Could you check a few things on this model? Use its own coordinates, in mm. A direction names the side the tool comes from. Round coordinates to 2 decimals unless told otherwise and drop trailing zeros. Order: outer loops, then holes, each group sorted by start corner. A loop starts at its lowest first (then second) coordinate and runs counter-clockwise, first axis right, second up. Notation, with made-up numbers: (79.5, 8.5) -> (104.5, 8.5) arc R15 ccw to (104.5, 18.5) -> close; hole circle Ø10 at (-38, 34). An arc over 180 degrees is marked (long way). One line per question, with ' | ' between items.
```python
from build123d import *

# Parameters (mm, degrees)
F0_W     = 7
F0_H     = 1.2
F2_W     = 50
F2_H     = 2
F3_DEPTH = 2.5


with BuildPart() as f1:
    # F0 (on Front) → F1 (revolve)
    with BuildSketch(Plane.XZ):
        Polygon((9, 6.694955), (7, 1.2), (7, 0), (7.763236, 0), (10.2, 6.694955), align=None)
        with Locations((3.5, 0.6)):
            Rectangle(F0_W, F0_H)
    revolve(axis=Axis((0, 0, 3.216552), (0, 0, -1)))

    # F2 (on Front) → F3 (join, symmetric)
    with BuildSketch(Plane.XZ):
        with Locations((34, 5.694955)):
            Rectangle(F2_W, F2_H)
    extrude(amount=F3_DEPTH, both=True)


solid = f1.part
```
1. On a 3-axis mill with a long thin cutter (end or side, diameter ignored), from which of +Z, -Z, +X, -X, +Y, -Y can I reach the whole of each face in a straight line? I mean faces 1 (the face through (34, 0, 4.695)), 2 (the face through (0, 0, 0)). Say none if no direction works.
From the geometry:
face 1: -Z, +X, +Y, -Y | face 2: -Z, +X, -X, +Y, -Y
2. I want a section at B-B on z = 2.25. List the corners of the cut face in (x, y) for me.
From the geometry:
outline: circle Ø17.16 at (0, 0); hole circle Ø14.76 at (0, 0)
3. I want a section at D-D on x = 33.5. List the corners of the cut face in (y, z) for me.
From the geometry:
outline: (-2.5, 4.69) -> (2.5, 4.69) -> (2.5, 6.69) -> (-2.5, 6.69) -> close
4. I'm going to push flat-ended pins straight in: pin 1 (1 mm diameter, centred on y = 6.5, z = 2, fed in from +X); pin 2 (2.5 mm diameter, centred on x = 39.5, y = 1, fed in from -Z); pin 3 (1 mm diameter, centred on x = 21.5, z = 5.5, fed in from +Y). Where does each tip first touch, or does it pass through?
From the geometry:
pin 1: stops at x = 6.07 | pin 2: stops at z = 4.69 | pin 3: stops at y = 2.5
5. I want a section at A-A on x = 0. List the corners of the cut face in (y, z) for me, and give its area (3 significant figures).
From the geometry:
outline: (-10.2, 6.69) -> (-7.76, 0) -> (7.76, 0) -> (10.2, 6.69) -> (9, 6.69) -> (7, 1.2) -> (-7, 1.2) -> (-9, 6.69) -> close | area: 32.3 mm²
6. I want a section at C-C on y = 0. List the corners of the cut face in (x, z) for me, and give its area (3 significant figures).
From the geometry:
outline: (-10.2, 6.69) -> (-7.76, 0) -> (7.76, 0) -> (9.47, 4.69) -> (59, 4.69) -> (59, 6.69) -> (9, 6.69) -> (7, 1.2) -> (-7, 1.2) -> (-9, 6.69) -> close | area: 131 mm²
7. I need wall thicknesses on probe 1 along Y at (x, z) = (45.5, 6.25); probe 2 along X at (y, z) = (1.25, 2.25); probe 3 along Y at (x, z) = (1.5, 2.75). Which ranges of each line are inside material? Lowest first, please.
From the geometry:
probe 1: y = -2.5 to 2.5 | probe 2: x = -8.49 to -7.28, 7.28 to 8.49 | probe 3: y = -8.63 to -7.41, 7.41 to 8.63
8. If we mould it in two halves opening along Y, with no side actions, what happens to faces 3 (the face through (0, 0, 1.2)), 4 (the face through (34, 2.5, 6)), 5 (the face through (59, 0, 6))? For each: pulls with the +Y half, pulls with the -Y half, needs draft (parallel to the pull), parting line crosses it, or undercut.
From the geometry:
face 3: undercut | face 4: pulls with the +Y half | face 5: needs draft
